Verification items for the finished model (mm, model axes). Face numbers are marked on the shaded views. A direction names the side the tool comes from. Coordinates: 2 decimals unless noted, no trailing zeros. Order: outer loops, then holes, each group sorted by start corner. A loop starts at its lowest first (then second) coordinate and runs counter-clockwise, first axis right, second up. Notation, with made-up numbers: (-26, 57.5) -> (-4, 57.5) arc R7 ccw to (-4, 70.5) -> close; hole circle Ø5 at (-25.5, 30.25). An arc over 180 degrees is marked (long way). Use CSV: the item, a comma, the result in double quotes. Start each with the question number.
1) Tool access check on the marked faces 1 and 2. Record the directions out of +Z, -Z, +X, -X, +Y, -Y that give a thin tool (end or side, any length) a straight path to the whole face; none if there is none.
2) Sectioned sample at B-B on x = 10. Record the boundary of the cut face in (y, z).
3) Scan lines: line 1 along Y through (x, z) = (10, 13); line 2 along Y through (x, z) = (10, -44.5); line 3 along X through (y, z) = (17, -78.5). Record each from-to range of solid material in increasing order.
4) Go/stop test with flat-tipped pins: pin 1 (1 mm diameter, centred on x = -5, z = -17.5, fed in from +Y); pin 2 (3 mm diameter, centred on y = 18, z = -62, fed in from -X); pin 3 (4.5 mm diameter, centred on x = 10, y = 8, fed in from -Z). Record where each tip stops, or that it passes through.
5) Sectioned sample at D-D on y = 16.75. Record the boundary of the cut face in (x, z), then the cut area to 3 significant figures.
6) Sectioned sample at C-C on z = -52. Record the boundary of the cut face in (x, y).
7) Sectioned sample at A-A on y = 10. Record the boundary of the cut face in (x, z), then the cut area to 4 significant figures.
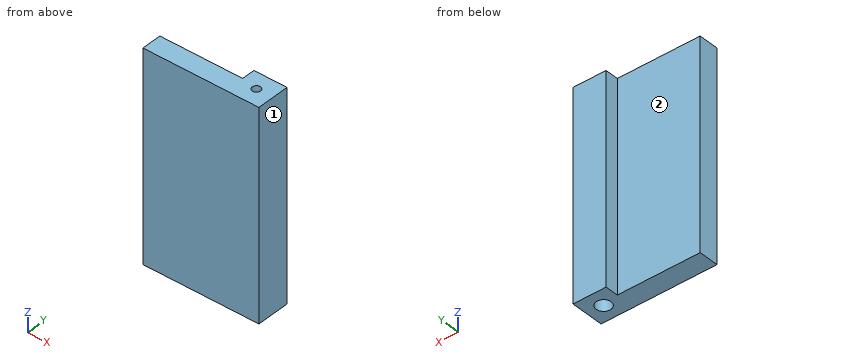
Autodesk Inventor part; units mm, degrees
ref_plane "YZ Plane" through (0, 0, 0) normal (1, 0, 0) x (0, 1, 0)
ref_plane "XZ Plane" through (0, 0, 0) normal (0, 1, 0) x (-1, 0, 0)
ref_plane "XY Plane" through (0, 0, 0) normal (0, 0, 1) x (1, 0, 0)
sketch "Sketch1" plane through (0, 0, 0) normal (0, 0, 1) x (1, 0, 0)
  line L0 (0, 20) -> (20, 20)
  line L1 (20, 20) -> (20, 0)
  line L2 (20, 0) -> (0, 0)
  line L3 (0, 0) -> (0, 20)
  circle A0 centre (10, 10) radius 2.5
  dimension "d0" = 20
  dimension "d1" = 20
  dimension "d5" = 10
  dimension "d6" = 10
  dimension "d7" = 5
extrude "Extrusion2" add sketch "Sketch1" along normal blind 25
sketch "Sketch3" plane through (0, 0, 0) normal (0, 0, -1) x (-1, 0, 0)
  line L0 (-20, 20) -> (0, 20)
  line L1 (0, 20) -> (0, 0)
  line L2 (-20, 20) -> (0, 20)
  line L3 (0, 20) -> (0, 0)
  line L4 (0, 0) -> (-20, 0)
  line L5 (-20, 0) -> (-20, 20)
  circle A0 centre (-10, 10) radius 4.5
  dimension "d10" = 9
extrude "Extrusion3" add sketch "Sketch3" along normal blind 100
sketch "Sketch4" plane through (0, 0, 25) normal (0, 0, 1) x (1, 0, 0)
  line L0 (0, 0) -> (20, 0)
  line L1 (0, 0) -> (-50, 0)
  line L2 (-50, 0) -> (-50, 12)
  line L3 (-50, 12) -> (0, 12)
  line L4 (0, 12) -> (0, 0)
  point P0 (0, 6)
  dimension "d13" = 12
  dimension "d14" = 50
extrude "Extrusion4" add sketch "Sketch4" against normal blind 125
equation "\"d1\" = d0"
properties part number "Touchscreen mount v04"
Answers follow:
1,face 1,"+Z, -Z, +X, +Y, -Y"
1,face 2,"+Z, -Z, -X, +Y"
2,outline,"(0, -100) -> (5.5, -100) -> (5.5, 0) -> (7.5, 0) -> (7.5, 25) -> (0, 25) -> close; (12.5, 0) -> (14.5, 0) -> (14.5, -100) -> (20, -100) -> (20, 25) -> (12.5, 25) -> close"
3,line 1,"y = 0 to 7.5, 12.5 to 20"
3,line 2,"y = 0 to 5.5, 14.5 to 20"
3,line 3,"x = 0 to 20"
4,pin 1,"stops at y = 12"
4,pin 2,"stops at x = 0"
4,pin 3,"stops at z = 0"
5,outline,"(0, -100) -> (20, -100) -> (20, 25) -> (0, 25) -> close"
5,area,"2,500 mm²"
6,outline,"(-50, 0) -> (20, 0) -> (20, 20) -> (0, 20) -> (0, 12) -> (-50, 12) -> close; hole circle Ø9 at (10, 10)"
7,outline,"(-50, -100) -> (5.5, -100) -> (5.5, 0) -> (7.5, 0) -> (7.5, 25) -> (-50, 25) -> close; (12.5, 0) -> (14.5, 0) -> (14.5, -100) -> (20, -100) -> (20, 25) -> (12.5, 25) -> close"
7,area,"7,725 mm²"
